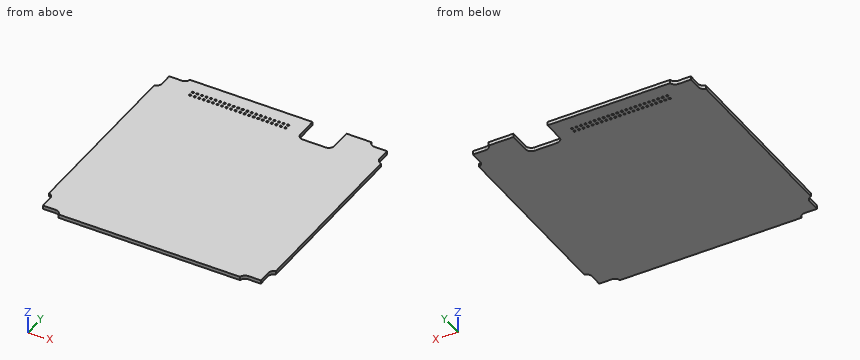
```python
from build123d import *

# Parameters (mm, degrees)
BOSS_EXTRUDE1_DEPTH = 1.5875
FILLET1_R           = 2.54
SKETCH2_R           = 0.45
CUT_EXTRUDE1_DEPTH  = 71.728496069
SKETCH3_W           = 15
SKETCH3_H           = 1.5875
CUT_EXTRUDE2_DEPTH  = 11.652
FILLET2_R           = 2.54


with BuildPart() as part:
    # Sketch1 → Boss-Extrude1 (new body)
    with BuildSketch(Plane.XY):
        Polygon((40, 50), (-40, 50), (-40, 48), (-48, 48), (-48, 40), (-50, 40), (-50, -37.864895224), (-50, -40), (-48, -40), (-48, -48), (-40, -48), (-40, -50), (-37.864895224, -50), (40, -50), (40, -48), (48, -48), (48, -40), (50, -40), (50, 40), (48, 40), (48, 48), (40, 48), align=None)
    extrude(amount=BOSS_EXTRUDE1_DEPTH)

    # Fillet1
    # the kernel refuses this fillet: 2.54 mm, written as the material it adds along each edge
    with BuildSketch(Plane(origin=(-48, -40, 0), x_dir=(0, -1, 0), z_dir=(0, 0, 1)), Plane(origin=(40, -48, 0), x_dir=(1, 0, 0), z_dir=(0, 0, 1)), Plane(origin=(48, 40, 0), x_dir=(0, 1, 0), z_dir=(0, 0, 1)), Plane(origin=(-40, 48, 0), x_dir=(-1, 0, 0), z_dir=(0, 0, 1))) as fillet1_piece_1:
        with BuildLine():
            CenterArc((2.481934729, -2.54), FILLET1_R, 90, 77.725329785)
            Line((0, -2), (-0.049638695, -1.9892))
            ThreePointArc((-0.049638695, -1.9892), (-0.0508, -1), (-0.0508, 0))
            Line((-0.0508, 0), (0, 0.0508))
            Line((0, 0.0508), (2.481934729, 0.0508))
            Line((2.481934729, 0.0508), (2.481934729, 0))
        make_face()
    extrude(amount=1.5875)
    with BuildSketch(Plane(origin=(-40, -48, 0), x_dir=(-3.737454790095179e-12, -1.0, 0), z_dir=(0, 0, 1)), Plane(origin=(48, -40, 0), x_dir=(1.0, -3.7339020764163554e-12, 0), z_dir=(0, 0, 1)), Plane(origin=(-48, 40, 0), x_dir=(-1.0, 3.737454790095126e-12, 0), z_dir=(0, 0, 1))) as fillet1_piece_2:
        with BuildLine():
            CenterArc((2.54, -2.481934729), FILLET1_R, 102.274670215, 77.725329785)
            Line((0, -2.481934729), (-0.0508, -2.481934729))
            Line((-0.0508, -2.481934729), (-0.0508, 0))
            Line((-0.0508, 0), (0, 0.0508))
            ThreePointArc((0, 0.0508), (1, 0.0508), (1.9892, 0.049638695))
            Line((1.9892, 0.049638695), (2, 0))
        make_face()
    extrude(amount=1.5875)
    with BuildSketch(Plane(origin=(40, 48, 0), x_dir=(1, 0, 0), z_dir=(0, 0, 1))) as fillet1_piece_3:
        with BuildLine():
            CenterArc((2.481934729, 2.54), FILLET1_R, 192.274670215, 77.725329785)
            Line((0, 2), (-0.049638695, 1.9892))
            ThreePointArc((-0.049638695, 1.9892), (-0.0508, 1), (-0.0508, 0))
            Line((-0.0508, 0), (0, -0.0508))
            Line((0, -0.0508), (2.481934729, -0.0508))
            Line((2.481934729, -0.0508), (2.481934729, 0))
        make_face()
    extrude(amount=1.5875)

    # Sketch2 → Cut-Extrude1 (cut, through all)
    with BuildSketch(Plane.XY.offset(1.5875)):
        with Locations((-35, 43.55)):
            Circle(SKETCH2_R)
        with Locations((-33, 43.55)):
            Circle(SKETCH2_R)
        with Locations((-31, 43.55)):
            Circle(SKETCH2_R)
        with Locations((-29, 43.55)):
            Circle(SKETCH2_R)
        with Locations((-27, 43.55)):
            Circle(SKETCH2_R)
        with Locations((-25, 43.55)):
            Circle(SKETCH2_R)
        with Locations((-23, 43.55)):
            Circle(SKETCH2_R)
        with Locations((-21, 43.55)):
            Circle(SKETCH2_R)
        with Locations((-19, 43.55)):
            Circle(SKETCH2_R)
        with Locations((-17, 43.55)):
            Circle(SKETCH2_R)
        with Locations((-15, 43.55)):
            Circle(SKETCH2_R)
        with Locations((-13, 43.55)):
            Circle(SKETCH2_R)
        with Locations((-11, 43.55)):
            Circle(SKETCH2_R)
        with Locations((-9, 43.55)):
            Circle(SKETCH2_R)
        with Locations((-7, 43.55)):
            Circle(SKETCH2_R)
        with Locations((-5, 43.55)):
            Circle(SKETCH2_R)
        with Locations((-3, 43.55)):
            Circle(SKETCH2_R)
        with Locations((-1, 43.55)):
            Circle(SKETCH2_R)
        with Locations((1, 43.55)):
            Circle(SKETCH2_R)
        with Locations((3, 43.55)):
            Circle(SKETCH2_R)
        with Locations((5, 43.55)):
            Circle(SKETCH2_R)
        with Locations((7, 43.55)):
            Circle(SKETCH2_R)
        with Locations((-33, 41.55)):
            Circle(SKETCH2_R)
        with Locations((-31, 41.55)):
            Circle(SKETCH2_R)
        with Locations((-29, 41.55)):
            Circle(SKETCH2_R)
        with Locations((-27, 41.55)):
            Circle(SKETCH2_R)
        with Locations((-25, 41.55)):
            Circle(SKETCH2_R)
        with Locations((-23, 41.55)):
            Circle(SKETCH2_R)
        with Locations((-21, 41.55)):
            Circle(SKETCH2_R)
        with Locations((-19, 41.55)):
            Circle(SKETCH2_R)
        with Locations((-17, 41.55)):
            Circle(SKETCH2_R)
        with Locations((-15, 41.55)):
            Circle(SKETCH2_R)
        with Locations((-13, 41.55)):
            Circle(SKETCH2_R)
        with Locations((-11, 41.55)):
            Circle(SKETCH2_R)
        with Locations((-9, 41.55)):
            Circle(SKETCH2_R)
        with Locations((-7, 41.55)):
            Circle(SKETCH2_R)
        with Locations((-5, 41.55)):
            Circle(SKETCH2_R)
        with Locations((-3, 41.55)):
            Circle(SKETCH2_R)
        with Locations((-1, 41.55)):
            Circle(SKETCH2_R)
        with Locations((1, 41.55)):
            Circle(SKETCH2_R)
        with Locations((3, 41.55)):
            Circle(SKETCH2_R)
        with Locations((5, 41.55)):
            Circle(SKETCH2_R)
        with Locations((7, 41.55)):
            Circle(SKETCH2_R)
        with Locations((-35, 41.55)):
            Circle(SKETCH2_R)
    extrude(amount=-CUT_EXTRUDE1_DEPTH, mode=Mode.SUBTRACT)

    # Sketch3 → Cut-Extrude2 (cut)
    with BuildSketch(Plane(origin=(0, 50, 0), x_dir=(1, 0, 0), z_dir=(0, 1, 0))):
        with Locations((21.5125, -0.79375)):
            Rectangle(SKETCH3_W, SKETCH3_H)
    extrude(amount=-CUT_EXTRUDE2_DEPTH, mode=Mode.SUBTRACT)

    # Fillet2
    fillet2_edges = [part.edges().sort_by_distance(p)[0] for p in [
        (14.0125, 38.348, 0.79375),
        (29.0125, 38.348, 0.79375),
    ]]
    fillet(fillet2_edges, radius=FILLET2_R)


solid = part.part
```
Part model, mm, in its own coordinate system. Round coordinates to 2 decimals unless told otherwise and drop trailing zeros. Answer in a Markdown table with one row per item. Add a question column.
Q1. Wall check: L1, parallel to Y at x = -31, z = 1.25; L2, parallel to Y at x = -42.5, z = 0.85. Give the ranges that are in metal, low to high. Write a range as from..to.
Q2. Cut at A-A on z = 0.4. Give the number of separate pieces and of enclosed holes in the cut face, and give its area (3 significant figures).
Q3. Pin check, flat tips, straight feed: pin 1 (0.5 mm diameter, centred on x = -45.5, z = 0.5, fed in from -Y); pin 2 (0.8 mm diameter, centred on y = 45, z = 1, fed in from -X); pin 3 (0.5 mm diameter, centred on x = -45, z = 1, fed in from +Y). Stop position of each tip, or through.
Established:
| question | item | result |
|---|---|---|
| 1 | L1 | y = -50..41.1, 42..43.1, 44..50 |
| 1 | L2 | y = -48..48 |
| 2 | separate pieces | 1 |
| 2 | enclosed holes | 44 |
| 2 | area | 9,670 mm2 |
| 3 | pin 1 | stops at y = -48 |
| 3 | pin 2 | stops at x = -48 |
| 3 | pin 3 | stops at y = 48 |
